Model file for the job. Use its own axes, mm. A direction names the side the tool comes from. Round coordinates to 2 decimals unless told otherwise and drop trailing zeros. Loops run counter-clockwise (first coordinate to the right, second up) from the corner with the lowest first, then second, coordinate; pieces in that order, holes last. Notation, with made-up numbers: (-8.5, 5) -> (7.5, 5) arc R10 ccw to (7.5, 20) -> close; hole circle Ø7 at (56.25, -21.5). An arc over 180 degrees is marked (long way). Use a Markdown table: item, result. Add a question column.
```python
from build123d import *

# Parameters (mm, degrees)
MODEL_R                 = 1.5
SALIENTE_EXTRUIR1_DEPTH = 3


with BuildPart() as part:
    # Model → Saliente-Extruir1 (new body)
    with BuildSketch(Plane.XY):
        with BuildLine():
            Line((213.25077615, 152.428489513), (213.25077615, 170.428489513))
            ThreePointArc((213.25077615, 170.428489513), (208.75077615, 174.928489513), (204.25077615, 170.428489513))
            Line((204.25077615, 170.428489513), (204.25077615, 152.428489513))
            ThreePointArc((204.25077615, 152.428489513), (208.75077615, 147.928489513), (213.25077615, 152.428489513))
        make_face()
        with Locations((208.75077615, 152.428489513)):
            Circle(MODEL_R, mode=Mode.SUBTRACT)
        with Locations((208.75077615, 170.428489513)):
            Circle(MODEL_R, mode=Mode.SUBTRACT)
        with BuildLine():
            Line((207.12577615, 158.928489513), (207.12577615, 163.928489513))
            ThreePointArc((207.12577615, 163.928489513), (207.345446064, 164.458819599), (207.87577615, 164.678489513))
            Line((207.87577615, 164.678489513), (209.62577615, 164.678489513))
            ThreePointArc((209.62577615, 164.678489513), (210.156106235, 164.458819599), (210.37577615, 163.928489513))
            Line((210.37577615, 163.928489513), (210.37577615, 158.928489513))
            ThreePointArc((210.37577615, 158.928489513), (210.156106235, 158.398159427), (209.62577615, 158.178489513))
            Line((209.62577615, 158.178489513), (207.87577615, 158.178489513))
            ThreePointArc((207.87577615, 158.178489513), (207.345446064, 158.398159427), (207.12577615, 158.928489513))
        make_face(mode=Mode.SUBTRACT)
    extrude(amount=SALIENTE_EXTRUIR1_DEPTH)


solid = part.part
```
1) Cut at C-C on x = 209.25. Write the cut outline in (y, z), and give its area (3 significant figures).
2) Tool access for faces 1 (the face through (209, 158.178, 1)), 2 (the face through (208.85, 174.927, 1.479)): list every direction of +Z, -Z, +X, -X, +Y, -Y with a clear straight run to the whole face (end or side of a thin tool).
3) Wall check: probe 1 along Y at (x, z) = (208.75, 2.75); probe 2 along Y at (x, z) = (208, 1.7); probe 3 along X at (y, z) = (160.5, 0.75). Give the ranges that are in metal, low to high. Write a range as from..to.
4) Pull direction X, two halves, no side cores. Call faces 3 (the face through (208.65, 147.93, 1.48)), 4 (the face through (204.251, 162, 1)), 5 (the face through (209, 164.678, 1)): +X half, -X half, draft (parallel to the pull), parting line (faces both ways), or undercut.
5) Cut at B-B on z = 1.7. Write the cut outline in (x, y).
6) Cut at A-A on y = 160. Write the cut outline in (x, z).
7) Cut at D-D on y = 169.25. Write the cut outline in (x, z), and give its area (3 significant figures).
Established:
| question | item | result |
|---|---|---|
| 1 | outline | (147.96, 0) -> (151.01, 0) -> (151.01, 3) -> (147.96, 3) -> close; (153.84, 0) -> (158.18, 0) -> (158.18, 3) -> (153.84, 3) -> close; (164.68, 0) -> (169.01, 0) -> (169.01, 3) -> (164.68, 3) -> close; (171.84, 0) -> (174.9, 0) -> (174.9, 3) -> (171.84, 3) -> close |
| 1 | area | 44.4 mm^2 |
| 2 | face 1 | +Z, -Z |
| 2 | face 2 | +Z, -Z, +Y |
| 3 | probe 1 | y = 147.93..150.93, 153.93..158.18, 164.68..168.93, 171.93..174.93 |
| 3 | probe 2 | y = 147.99..151.13, 153.73..158.18, 164.68..169.13, 171.73..174.87 |
| 3 | probe 3 | x = 204.25..207.13, 210.38..213.25 |
| 4 | face 3 | parting line |
| 4 | face 4 | -X half |
| 4 | face 5 | undercut |
| 5 | outline | (204.25, 152.43) arc R4.5 ccw to (213.25, 152.43) -> (213.25, 170.43) arc R4.5 ccw to (204.25, 170.43) -> close; hole (207.13, 158.93) arc R0.75 ccw to (207.88, 158.18) -> (209.63, 158.18) arc R0.75 ccw to (210.38, 158.93) -> (210.38, 163.93) arc R0.75 ccw to (209.63, 164.68) -> (207.88, 164.68) arc R0.75 ccw to (207.13, 163.93) -> close; hole circle Ø3 at (208.75, 152.43); hole circle Ø3 at (208.75, 170.43) |
| 6 | outline | (204.25, 0) -> (207.13, 0) -> (207.13, 3) -> (204.25, 3) -> close; (210.38, 0) -> (213.25, 0) -> (213.25, 3) -> (210.38, 3) -> close |
| 7 | outline | (204.25, 0) -> (207.82, 0) -> (207.82, 3) -> (204.25, 3) -> close; (209.68, 0) -> (213.25, 0) -> (213.25, 3) -> (209.68, 3) -> close |
| 7 | area | 21.4 mm^2 |
